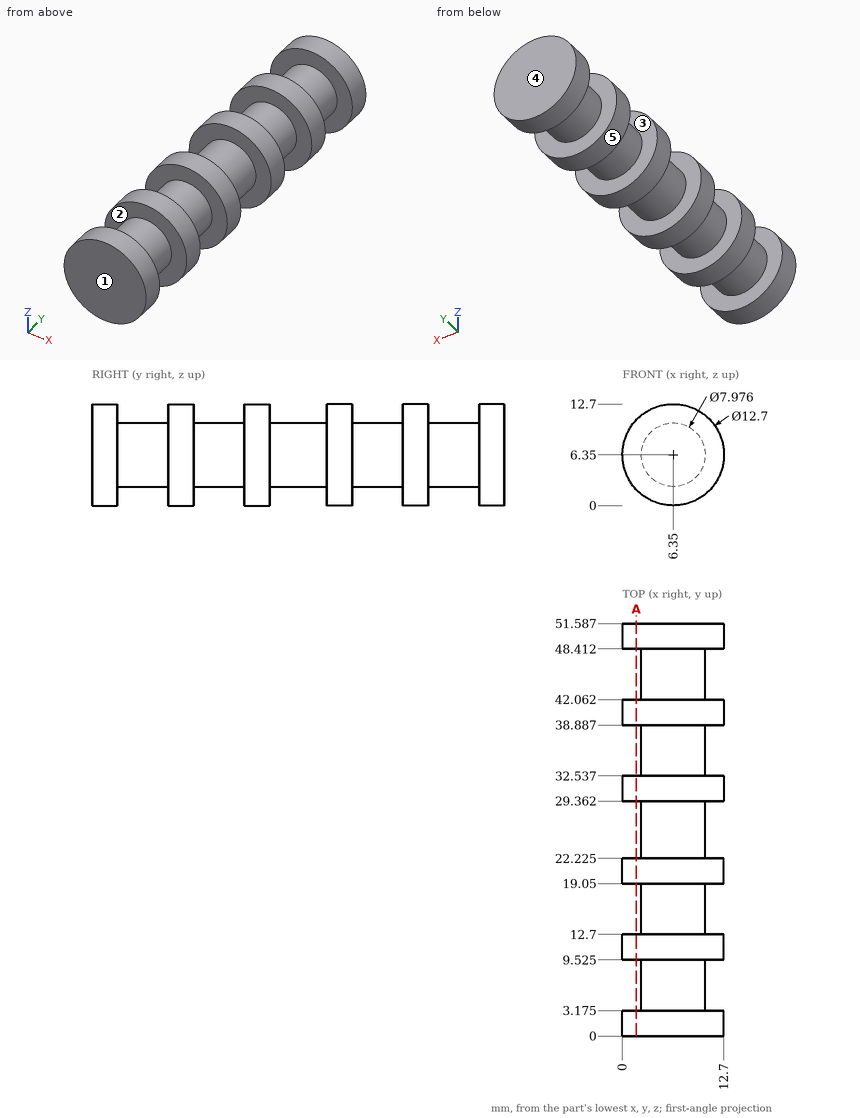
Could you check a few things on this drawing? It's one solid part, dimensions in mm from its lowest x, y, z. A direction names the side the tool comes from. Coordinates: 2 decimals unless noted, no trailing zeros. Write item = value, one per line.
1) Please list where these lines run through material, in increasing order: line 1 (Z direction, x = 6.25, y = 8); line 2 (Z direction, x = 4, y = 43); line 3 (X direction, y = 42.5, z = 3) (1 decimal). Write a range as [from, to].
Result set:
line_1 = [2.36, 10.34]
line_2 = [3.13, 9.57]
line_3 = [4.2, 8.5]
2) We'd pull the mould along Y, two halves only. Please class the marked faces 3, 4 and 5: +Y half, -Y half, draft (parallel to the pull), parting line (faces both ways), or undercut.
Result set:
face_3 = undercut
face_4 = +Y half
face_5 = draft
3) Suppose I cut it at A-A on x = 1.75. State how many separate pieces and enclosed holes the cut face has, plus the area to 3 significant figures.
Result set:
separate_pieces = 6
enclosed_holes = 0
area = 167 mm2
4) For the marked faces 1 and 2, which set-ups out of +Z, -Z, +X, -X, +Y, -Y let a thin tool reach every point of the face, with its end or its side?
Result set:
face_1 = +Z, -Z, +X, -X, -Y
face_2 = none
5) Will these pins go through, and if not, where does the flat tip stop? pin 1 Ø1 at (y, z) = (7, 3.5) entering from +X; pin 2 Ø3 at (y, z) = (38.5, 10) entering from +X; pin 3 Ø2 at (y, z) = (45, 5.5) entering from -X.
Result set:
pin_1 = 9.57
pin_2 = 12.31
pin_3 = 2.36
